```python
from build123d import *

# Parameters (mm, degrees)
BOSS_EXTRUDE1_DEPTH = 160
SKETCH2_R           = 4
SKETCH2_R_2         = 1.85
CUT_EXTRUDE1_DEPTH  = 33
SKETCH3_R           = 4
SKETCH3_R_2         = 1.85
CUT_EXTRUDE2_DEPTH  = 33
FILLET1_R           = 2


with BuildPart() as part:
    # Sketch1 → Boss-Extrude1 (new body)
    with BuildSketch(Plane.XY):
        Polygon((14, -16), (16, -16), (16, 16), (-16, 16), (-16, -16), (-14, -16), (-14, 14), (14, 14), align=None)
    extrude(amount=-BOSS_EXTRUDE1_DEPTH)

    # Sketch2 → Cut-Extrude1 (cut, through all)
    with BuildSketch(Plane(origin=(0, 16, 0), x_dir=(1, 0, 0), z_dir=(0, 1, 0))):
        with Locations((0, 32)):
            Circle(SKETCH2_R)
        with Locations((0, 64)):
            Circle(SKETCH2_R)
        with Locations((-0.175415159, 96)):
            Circle(SKETCH2_R)
        with Locations((0, 128)):
            Circle(SKETCH2_R)
        with Locations((0, 48)):
            Circle(SKETCH2_R)
        with Locations((0, 56)):
            Circle(SKETCH2_R_2)
        with Locations((0, 40)):
            Circle(SKETCH2_R_2)
        with Locations((8, 48)):
            Circle(SKETCH2_R_2)
        with Locations((-8, 48)):
            Circle(SKETCH2_R_2)
        with Locations((0, 24)):
            Circle(SKETCH2_R_2)
        with Locations((8, 16)):
            Circle(SKETCH2_R_2)
        with Locations((0, 16)):
            Circle(SKETCH2_R)
        with Locations((-8, 16)):
            Circle(SKETCH2_R_2)
        with Locations((-5.66, 10.34)):
            Circle(SKETCH2_R_2)
        with Locations((5.66, 10.34)):
            Circle(SKETCH2_R_2)
        with Locations((0, 8)):
            Circle(SKETCH2_R_2)
        with Locations((-5.66, 21.66)):
            Circle(SKETCH2_R_2)
        with Locations((5.66, 21.66)):
            Circle(SKETCH2_R_2)
        with Locations((0, 112)):
            Circle(SKETCH2_R)
        with Locations((0, 120)):
            Circle(SKETCH2_R_2)
        with Locations((0, 104)):
            Circle(SKETCH2_R_2)
        with Locations((8, 112)):
            Circle(SKETCH2_R_2)
        with Locations((-8, 112)):
            Circle(SKETCH2_R_2)
        with Locations((0, 88)):
            Circle(SKETCH2_R_2)
        with Locations((8, 80)):
            Circle(SKETCH2_R_2)
        with Locations((0, 80)):
            Circle(SKETCH2_R)
        with Locations((-8, 80)):
            Circle(SKETCH2_R_2)
        with Locations((-5.66, 74.34)):
            Circle(SKETCH2_R_2)
        with Locations((5.66, 74.34)):
            Circle(SKETCH2_R_2)
        with Locations((0, 72)):
            Circle(SKETCH2_R_2)
        with Locations((-5.66, 85.66)):
            Circle(SKETCH2_R_2)
        with Locations((5.66, 85.66)):
            Circle(SKETCH2_R_2)
        with Locations((0, 136)):
            Circle(SKETCH2_R_2)
        with Locations((-8, 144)):
            Circle(SKETCH2_R_2)
        with Locations((0, 144)):
            Circle(SKETCH2_R)
        with Locations((8, 144)):
            Circle(SKETCH2_R_2)
        with Locations((5.66, 149.66)):
            Circle(SKETCH2_R_2)
        with Locations((-5.66, 149.66)):
            Circle(SKETCH2_R_2)
        with Locations((0, 152)):
            Circle(SKETCH2_R_2)
        with Locations((5.66, 138.34)):
            Circle(SKETCH2_R_2)
        with Locations((-5.66, 138.34)):
            Circle(SKETCH2_R_2)
    extrude(amount=-CUT_EXTRUDE1_DEPTH, mode=Mode.SUBTRACT)

    # Sketch3 → Cut-Extrude2 (cut, through all)
    with BuildSketch(Plane(origin=(16, 0, 0), x_dir=(0, 0, -1), z_dir=(1, 0, 0))):
        with Locations((32, 0)):
            Circle(SKETCH3_R)
        with Locations((64, 0)):
            Circle(SKETCH3_R)
        with Locations((96, 0.175415159)):
            Circle(SKETCH3_R)
        with Locations((128, 0)):
            Circle(SKETCH3_R)
        with Locations((48, 0)):
            Circle(SKETCH3_R)
        with Locations((56, 0)):
            Circle(SKETCH3_R_2)
        with Locations((40, 0)):
            Circle(SKETCH3_R_2)
        with Locations((48, -8)):
            Circle(SKETCH3_R_2)
        with Locations((48, 8)):
            Circle(SKETCH3_R_2)
        with Locations((24, 0)):
            Circle(SKETCH3_R_2)
        with Locations((16, -8)):
            Circle(SKETCH3_R_2)
        with Locations((16, 0)):
            Circle(SKETCH3_R)
        with Locations((16, 8)):
            Circle(SKETCH3_R_2)
        with Locations((10.34, 5.66)):
            Circle(SKETCH3_R_2)
        with Locations((10.34, -5.66)):
            Circle(SKETCH3_R_2)
        with Locations((8, 0)):
            Circle(SKETCH3_R_2)
        with Locations((21.66, 5.66)):
            Circle(SKETCH3_R_2)
        with Locations((21.66, -5.66)):
            Circle(SKETCH3_R_2)
        with Locations((112, 0)):
            Circle(SKETCH3_R)
        with Locations((120, 0)):
            Circle(SKETCH3_R_2)
        with Locations((104, 0)):
            Circle(SKETCH3_R_2)
        with Locations((112, -8)):
            Circle(SKETCH3_R_2)
        with Locations((112, 8)):
            Circle(SKETCH3_R_2)
        with Locations((88, 0)):
            Circle(SKETCH3_R_2)
        with Locations((80, -8)):
            Circle(SKETCH3_R_2)
        with Locations((80, 0)):
            Circle(SKETCH3_R)
        with Locations((80, 8)):
            Circle(SKETCH3_R_2)
        with Locations((74.34, 5.66)):
            Circle(SKETCH3_R_2)
        with Locations((74.34, -5.66)):
            Circle(SKETCH3_R_2)
        with Locations((72, 0)):
            Circle(SKETCH3_R_2)
        with Locations((85.66, 5.66)):
            Circle(SKETCH3_R_2)
        with Locations((85.66, -5.66)):
            Circle(SKETCH3_R_2)
        with Locations((136, 0)):
            Circle(SKETCH3_R_2)
        with Locations((144, 8)):
            Circle(SKETCH3_R_2)
        with Locations((144, 0)):
            Circle(SKETCH3_R)
        with Locations((144, -8)):
            Circle(SKETCH3_R_2)
        with Locations((149.66, -5.66)):
            Circle(SKETCH3_R_2)
        with Locations((149.66, 5.66)):
            Circle(SKETCH3_R_2)
        with Locations((152, 0)):
            Circle(SKETCH3_R_2)
        with Locations((138.34, -5.66)):
            Circle(SKETCH3_R_2)
        with Locations((138.34, 5.66)):
            Circle(SKETCH3_R_2)
    extrude(amount=-CUT_EXTRUDE2_DEPTH, mode=Mode.SUBTRACT)

    # Fillet1
    fillet1_edges = [part.edges().sort_by_distance(p)[0] for p in [
        (-15, -16, -160),
        (-16, 16, -80),
        (16, 16, -80),
        (15, -16, -160),
        (15, -16, 0),
        (-15, -16, 0),
    ]]
    fillet(fillet1_edges, radius=FILLET1_R)


solid = part.part
```
Geometry: final body of the model. Coordinates: model frame, mm. Coordinates: 2 decimals unless noted, no trailing zeros. Write each loop counter-clockwise with the first axis right and the second up, starting at its lowest first coordinate (ties: lowest second). Pieces come first, ordered by that corner, then holes. Notation, with made-up numbers: M 18.25,14.25 L 23.25,14.25 A26 cw 23.25,39.25 Z; hole C 42,71 d1. An arc over 180 degrees is marked long. Use CSV: the item, a comma, the result in double quotes. Start each with the question number.
1. Cut plane D-D on z = -48. Count the separate pieces of the cut face and the enclosed holes in it, plus the area to 3 significant figures.
2. Cut plane C-C on x = -11.5. Return the cut outline in (y, z).
3. First-contact query: P1, Ø3.5, axis at y = -8, z = -48, coming from the -X side; P2, Ø1.5, axis at x = -12, z = -113, coming from the -Y side. Flat tips, straight axial feed; report the tip coordinate or a pass-through.
4. Mould query, pull axis Y, two halves, no side actions, for faces 1 (the face through (-0.401, 15.014, -70.194)), 2 (the face through (-14.99, 5.74, -136.49)). Classes: pulls with the +Y half, pulls with the -Y half, needs draft (parallel to the pull), parting line crosses it, or undercut.
5. Cut plane A-A on z = -32. Return the cut outline in (x, y).
6. Cut plane B-B on y = -12. Return the cut outline in (x, z), plus the area to 3 significant figures.
7. Ray query, probe 1 along Z at (x, y) = (-8, 15); probe 2 along X at (y, z) = (7, -109.5); probe 3 along Y at (x, z) = (15.2, -74.34). Return the intervals inside material, ascending.
Entries:
1,separate pieces,"10"
1,enclosed holes,"0"
1,area,"89.9 mm²"
2,outline,"M 14,-160 L 16,-160 L 16,0 L 14,0 Z"
3,P1,"through"
3,P2,"y = 14"
4,face 1,"needs draft"
4,face 2,"undercut"
5,outline,"M -16,-16 L -14,-16 L -14,-4 L -16,-4 Z; M -16,4 L -14,4 L -14,14 L -4,14 L -4,16 L -14,16 A2 ccw -16,14 Z; M 4,14 L 14,14 L 14,4 L 16,4 L 16,14 A2 ccw 14,16 L 4,16 Z; M 14,-16 L 16,-16 L 16,-4 L 14,-4 Z"
6,outline,"M -16,-160 L -14,-160 L -14,0 L -16,0 Z; M 14,-160 L 16,-160 L 16,0 L 14,0 Z"
6,area,"640 mm²"
7,probe 1,"-160 to -145.85, -142.15 to -113.85, -110.15 to -81.85, -78.15 to -49.85, -46.15 to -17.85, -14.15 to 0"
7,probe 2,"-16 to -14, 14 to 16"
7,probe 3,"-16 to -7.51, -3.81 to 3.81, 7.51 to 15.6"
